Input: part model. Units: mm. Frame: model coordinates. A direction names the side the tool comes from. Give positions to 0.01 mm unless a question says otherwise; leave off trailing zeros. Loops run counter-clockwise (first coordinate to the right, second up) from the corner with the lowest first, then second, coordinate; pieces in that order, holes last. Notation, with made-up numbers: (-37.5, 83) - (10.5, 83) arc R17 cw to (10.5, 102) - close; hole circle Ø1 at (27, 69.25). An arc over 180 degrees is marked (long way). One line per item, written item: value.
Autodesk Inventor part; units mm, degrees
ref_plane "作業平面1" through (0, 0, 0) normal (0, 0, 1) x (1, 0, 0)
ref_plane "YZ Plane" through (0, 0, 0) normal (1, 0, 0) x (0, 1, 0)
ref_plane "XZ Plane" through (0, 0, 0) normal (0, 1, 0) x (-1, 0, 0)
ref_plane "作業平面1" through (0, 0, 0) normal (0, 0, 1) x (1, 0, 0)
sketch "スケッチ2" plane through (0, 0, 0) normal (0, 0, 1) x (1, 0, 0)
  line L0 (0, 0) -> (7.35, 0) construction
  line L1 (7.35, 0) -> (7.35, 50) construction
  line L2 (0, 50) -> (7.35, 50) construction
  line L3 (0, 0) -> (0, 50) construction
  line L4 (-0.5, 0) -> (-0.5, 50) construction
  line L5 (19.5, 0) -> (19.5, 50) construction
  line L6 (139.5, 0) -> (139.5, -3) construction
  line L7 (139.5, 0) -> (4.5, 0) construction
  line L8 (4.5, -3) -> (4.5, 0) construction
  line L9 (139.5, -3) -> (4.5, -3) construction
  line L10 (139.5, 53) -> (139.5, 50) construction
  line L11 (4.5, 53) -> (139.5, 53) construction
  line L12 (4.5, 50) -> (4.5, 53) construction
  line L13 (4.5, 50) -> (139.5, 50) construction
  line L14 (-0.632, 5) -> (-130.632, 5) construction
  line L15 (-0.632, 45) -> (-130.632, 45) construction
  line L16 (-40.5, 10) -> (-40.5, 40)
  line L17 (-40.5, 40) -> (-0.5, 40)
  line L18 (-0.5, 40) -> (-0.5, 5)
  circle A0 centre (14.5, 15) radius 3.3
  circle A1 centre (14.5, 35) radius 3.3
  circle A2 centre (-30.5, 25) radius 3.3
  circle A3 centre (-10.5, 25) radius 3.3
  line L19 (-40.5, 10) -> (-0.5, 10)
  line L20 (-0.5, 0) -> (29.5, 0)
  line L21 (29.5, 0) -> (29.5, 50)
  line L22 (29.5, 50) -> (-0.5, 50)
  line L23 (-0.5, 50) -> (-0.5, 0)
  point P0 (9.5, 35)
  point P1 (-0.5, 40)
  point P2 (-0.5, 5)
  dimension "d1" = 40
  dimension "d2" = 30
  dimension "d4" = 50
  dimension "d5" = 15
  dimension "d13" = 6.6
  dimension "d17" = 6.6
  dimension "d19" = 10
  dimension "d20" = 6.6
  dimension "d22" = 10
  dimension "d23" = 6.6
  dimension "d25" = 15
  dimension "d27" = 10
  dimension "d29" = 15
  dimension "d30" = 15
  dimension "d31" = 30
  dimension "d32" = 50
  dimension "d33" = 15
  dimension "d34" = 15
extrude "押し出し1" add sketch "スケッチ2" along normal blind 3
fillet "フィレット1" radius 5 6 edges at (-40.5, 10, 1.5) (-40.5, 40, 1.5) (-0.5, 0, 1.5) (29.5, 0, 1.5) (-0.5, 50, 1.5) (29.5, 50, 1.5)
equation "\"d22\" = d19"
equation "\"d23\" = d13"
equation "\"d27\" = -0.5 * d2 + 0.5 * d28"
equation "\"d29\" = 0.5 * d2"
equation "\"d30\" = d29"
equation "\"d33\" = 0.5 * d31"
equation "\"d34\" = d33"
properties part number "bogie_mount" material "アルミニウム 6061"
Item 1: Access query for faces 1 (the face through (-0.5, 8, 1)), 2 (the face through (-40.5, 25, 1)). Directions: +Z, -Z, +X, -X, +Y, -Y. A direction counts if a zero-diameter tool reaches every point of the face in a straight line with its end or side. Return the directions, or none.
Verdict:
face 1: +Z, -Z, -X, -Y
face 2: +Z, -Z, -X, +Y, -Y
Item 2: Material intervals for L1, parallel to Y at x = 14.5, z = 1.65; L2, parallel to Y at x = -30.5, z = 1.3; L3, parallel to Y at x = 12.5, z = 1.1, sorted ascending.
Verdict:
L1: y = 0 to 11.7, 18.3 to 31.7, 38.3 to 50
L2: y = 10 to 21.7, 28.3 to 40
L3: y = 0 to 12.38, 17.62 to 32.38, 37.62 to 50
Item 3: Section C-C, the plane y = 25. Output: boundary loops of the cut face in (x, z).
Verdict:
outline: (-40.5, 0) - (-33.8, 0) - (-33.8, 3) - (-40.5, 3) - close; (-27.2, 0) - (-13.8, 0) - (-13.8, 3) - (-27.2, 3) - close; (-7.2, 0) - (29.5, 0) - (29.5, 3) - (-7.2, 3) - close
Item 4: Section A-A, the plane x = -10.5. Output: boundary loops of the cut face in (y, z), and give its area (3 significant figures).
Verdict:
outline: (10, 0) - (21.7, 0) - (21.7, 3) - (10, 3) - close; (28.3, 0) - (40, 0) - (40, 3) - (28.3, 3) - close
area: 70.2 mm^2
Item 5: Draft query along Y for faces 3 (the face through (14.07, 31.73, 1.48)), 4 (the face through (14, 0, 1)), 5 (the face through (-18, 40, 1)). Return one class per face: pulls with the +Y half, pulls with the -Y half, needs draft (parallel to the pull), parting line crosses it, or undercut.
Verdict:
face 3: undercut
face 4: pulls with the -Y half
face 5: pulls with the +Y half
Item 6: Section B-B, the plane z = 0.5. Output: boundary loops of the cut face in (x, y), and give its area (3 significant figures).
Verdict:
outline: (-40.5, 15) arc R5 ccw to (-35.5, 10) - (-0.5, 10) - (-0.5, 5) arc R5 ccw to (4.5, 0) - (24.5, 0) arc R5 ccw to (29.5, 5) - (29.5, 45) arc R5 ccw to (24.5, 50) - (4.5, 50) arc R5 ccw to (-0.5, 45) - (-0.5, 40) - (-35.5, 40) arc R5 ccw to (-40.5, 35) - close; hole circle Ø6.6 at (-30.5, 25); hole circle Ø6.6 at (-10.5, 25); hole circle Ø6.6 at (14.5, 15); hole circle Ø6.6 at (14.5, 35)
area: 2,530 mm^2
Item 7: Pin query (flat end, axial travel): P1, Ø0.9, axis at y = 42, z = 1, coming from the -X side; P2, Ø1.5, axis at x = -21, z = 1.5, coming from the -Y side. Return the tip coordinate at first contact, or that it passes through.
Verdict:
P1: stops at x = -0.5
P2: stops at y = 10
Item 8: Section D-D, the plane x = 14.5. Output: boundary loops of the cut face in (y, z).
Verdict:
outline: (0, 0) - (11.7, 0) - (11.7, 3) - (0, 3) - close; (18.3, 0) - (31.7, 0) - (31.7, 3) - (18.3, 3) - close; (38.3, 0) - (50, 0) - (50, 3) - (38.3, 3) - close
